Could you check a few things on this model? Use its own coordinates, in mm. A direction names the side the tool comes from. Round coordinates to 2 decimals unless told otherwise and drop trailing zeros. Write each loop counter-clockwise with the first axis right and the second up, starting at its lowest first coordinate (ties: lowest second). Pieces come first, ordered by that corner, then holes. Notation, with made-up numbers: (-21, 88) - (2, 88) arc R22 ccw to (2, 116) - close; hole circle Ø4 at (38, -12). An arc over 180 degrees is marked (long way). Write each question's results on one line, items separated by ' | '. Start each with the question number.
(1) Imagine slicing it at B-B on y = 24.5. Write out the boundary of the cut face in (x, z).
(2) Imagine slicing it at C-C on z = 0.5. Write out the boundary of the cut face in (x, y).
(3) Thinking about a two-plate mould opening in Y: for faces 4 (the flat face through (53, 82, 1)), 5 (the cylindrical face through (10.234, 71.195, 0.74)), 6 (the flat face through (109, 39, 1)), 7 (the flat face through (53, -2, 1)), which applies, +Y half, -Y half, draft (parallel to the pull), parting line (faces both ways), or undercut?
(4) Imagine slicing it at D-D on x = 37.5. Write out the boundary of the cut face in (y, z).
(5) Please list where these lines run through material, in increasing order: line 1 (Y direction, x = 11.04, z = 1.9); line 2 (X direction, y = 7.54, z = 1.9); line 3 (X direction, y = 58.5, z = 1.55). Write a range as [from, to].
(6) On a 3-axis mill with a long thin cutter (end or side, diameter ignored), from which of +Z, -Z, +X, -X, +Y, -Y can I reach the whole of each face in a straight line? I mean faces 1 (the flat face through (32, 5.8, 1)), 2 (the cylindrical face through (98.957, 7.408, 2.24)), 3 (the flat face through (-0.2, 40.2, 3)). Say none if no direction works.
(7) For P1, Ø3, axis at x = 97, y = 8, coming from the +Z side; P2, Ø2.5, axis at x = 11.04, y = 7.54, coming from the +Z side, each with a flat end and sliding along its axis, tell me the tip position at first contact or that it passes through.
(8) Imagine slicing it at A-A on x = 95.96. Write out the boundary of the cut face in (y, z), then the cut area to 3 significant figures.
```python
from build123d import *

# Parameters (mm, degrees)
SKETCH_9_W                                     = 111
SKETCH_9_H                                     = 84
BOTTOM_BASE_1P5MM_FULL_111X84_DEPTH            = 1.5
SKETCH_10_W                                    = 101
SKETCH_10_H                                    = 74
SKETCH_10_R                                    = 3
BOTTOM_CENTER_FULL_THICKNESS_EXCEPT_STAN_DEPTH = 3
SKETCH_11_W                                    = 111
SKETCH_11_H                                    = 2
BOTTOM_OUTER_FRONT_OVERHANG_FULL_3MM_DEPTH     = 3
SKETCH_12_W                                    = 111
SKETCH_12_H                                    = 2
BOTTOM_OUTER_REAR_OVERHANG_FULL_3MM_DEPTH      = 3
SKETCH_13_W                                    = 2
SKETCH_13_H                                    = 80
BOTTOM_OUTER_LEFT_OVERHANG_FULL_3MM_DEPTH      = 3
SKETCH_14_W                                    = 2
SKETCH_14_H                                    = 80
BOTTOM_OUTER_RIGHT_OVERHANG_FULL_3MM_DEPTH     = 3
SKETCH_16_R                                    = 1.5
BOTTOM_M3_THROUGH_3MM_DEPTH                    = 1.5
SKETCH_18_R                                    = 16.5
BOTTOM_BATTERY_THROUGH_CLEARANCE_DEPTH         = 3
SKETCH_20_W                                    = 23
SKETCH_20_H                                    = 23
BOTTOM_BUZZER_THROUGH_CUT_DEPTH                = 3


with BuildPart() as part:
    # Sketch 9 → bottom_base_1p5mm_full_111x84 (new body)
    with BuildSketch(Plane.XY):
        with Locations((53.5, 40)):
            Rectangle(SKETCH_9_W, SKETCH_9_H)
    extrude(amount=BOTTOM_BASE_1P5MM_FULL_111X84_DEPTH)

    # Sketch 10 → bottom_center_full_thickness_except_stan (add)
    with BuildSketch(Plane.XY):
        with Locations((53.5, 40)):
            Rectangle(SKETCH_10_W, SKETCH_10_H)
        with Locations(Location((11.04, 7.54, 0), (0, 0, 180))):
            Circle(SKETCH_10_R, mode=Mode.SUBTRACT)
        with Locations(Location((95.96, 7.54, 0), (0, 0, 180))):
            Circle(SKETCH_10_R, mode=Mode.SUBTRACT)
        with Locations(Location((11.04, 72.46, 0), (0, 0, 180))):
            Circle(SKETCH_10_R, mode=Mode.SUBTRACT)
        with Locations(Location((95.96, 72.46, 0), (0, 0, 180))):
            Circle(SKETCH_10_R, mode=Mode.SUBTRACT)
    extrude(amount=BOTTOM_CENTER_FULL_THICKNESS_EXCEPT_STAN_DEPTH)

    # Sketch 11 → bottom_outer_front_overhang_full_3mm (add)
    with BuildSketch(Plane.XY):
        with Locations((53.5, -1)):
            Rectangle(SKETCH_11_W, SKETCH_11_H)
    extrude(amount=BOTTOM_OUTER_FRONT_OVERHANG_FULL_3MM_DEPTH)

    # Sketch 12 → bottom_outer_rear_overhang_full_3mm (add)
    with BuildSketch(Plane.XY):
        with Locations((53.5, 81)):
            Rectangle(SKETCH_12_W, SKETCH_12_H)
    extrude(amount=BOTTOM_OUTER_REAR_OVERHANG_FULL_3MM_DEPTH)

    # Sketch 13 → bottom_outer_left_overhang_full_3mm (add)
    with BuildSketch(Plane.XY):
        with Locations((-1, 40)):
            Rectangle(SKETCH_13_W, SKETCH_13_H)
    extrude(amount=BOTTOM_OUTER_LEFT_OVERHANG_FULL_3MM_DEPTH)

    # Sketch 14 → bottom_outer_right_overhang_full_3mm (add)
    with BuildSketch(Plane.XY):
        with Locations((108, 40)):
            Rectangle(SKETCH_14_W, SKETCH_14_H)
    extrude(amount=BOTTOM_OUTER_RIGHT_OVERHANG_FULL_3MM_DEPTH)

    # Sketch 16 → bottom_m3_through_3mm (cut)
    with BuildSketch(Plane.XY):
        with Locations(Location((11.04, 7.54, 0), (0, 0, 180))):
            Circle(SKETCH_16_R)
        with Locations(Location((95.96, 7.54, 0), (0, 0, 180))):
            Circle(SKETCH_16_R)
        with Locations(Location((11.04, 72.46, 0), (0, 0, 180))):
            Circle(SKETCH_16_R)
        with Locations(Location((95.96, 72.46, 0), (0, 0, 180))):
            Circle(SKETCH_16_R)
    extrude(amount=BOTTOM_M3_THROUGH_3MM_DEPTH, mode=Mode.SUBTRACT)

    # Sketch 18 → bottom_battery_through_clearance (cut)
    with BuildSketch(Plane.XY):
        with Locations(Location((58.8, 24.5, 0), (0, 0, 180))):
            Circle(SKETCH_18_R)
    extrude(amount=BOTTOM_BATTERY_THROUGH_CLEARANCE_DEPTH, mode=Mode.SUBTRACT)

    # Sketch 20 → bottom_buzzer_through_cut (cut)
    with BuildSketch(Plane.XY):
        with Locations((32.4, 17.3)):
            Rectangle(SKETCH_20_W, SKETCH_20_H)
    extrude(amount=BOTTOM_BUZZER_THROUGH_CUT_DEPTH, mode=Mode.SUBTRACT)


solid = part.part
```
Response:
1) outline: (-2, 0) - (20.9, 0) - (20.9, 3) - (3, 3) - (3, 1.5) - (0, 1.5) - (0, 3) - (-2, 3) - close; (75.3, 0) - (109, 0) - (109, 3) - (107, 3) - (107, 1.5) - (104, 1.5) - (104, 3) - (75.3, 3) - close
2) outline: (-2, -2) - (109, -2) - (109, 82) - (-2, 82) - close; hole circle Ø3 at (11.04, 7.54); hole circle Ø3 at (11.04, 72.46); hole (20.9, 5.8) - (43.9, 5.8) - (43.9, 17.41) arc R16.5 ccw (long way) to (42.87, 28.8) - (20.9, 28.8) - close; hole circle Ø3 at (95.96, 7.54); hole circle Ø3 at (95.96, 72.46)
3) face 4: +Y half | face 5: undercut | face 6: draft | face 7: -Y half
4) outline: (-2, 0) - (5.8, 0) - (5.8, 3) - (3, 3) - (3, 1.5) - (0, 1.5) - (0, 3) - (-2, 3) - close; (28.8, 0) - (82, 0) - (82, 3) - (80, 3) - (80, 1.5) - (77, 1.5) - (77, 3) - (28.8, 3) - close
5) line 1: [-2, 0], [3, 4.54], [10.54, 69.46], [75.46, 77], [80, 82] | line 2: [-2, 0], [3, 8.04], [14.04, 20.9], [43.9, 92.96], [98.96, 104], [107, 109] | line 3: [-2, 0], [3, 104], [107, 109]
6) face 1: +Z, -Z | face 2: +Z | face 3: +Z, +X, -X, +Y, -Y
7) P1: z = 1.5 | P2: through
8) outline: (-2, 0) - (6.04, 0) - (6.04, 1.5) - (4.54, 1.5) - (4.54, 3) - (3, 3) - (3, 1.5) - (0, 1.5) - (0, 3) - (-2, 3) - close; (9.04, 0) - (70.96, 0) - (70.96, 1.5) - (69.46, 1.5) - (69.46, 3) - (10.54, 3) - (10.54, 1.5) - (9.04, 1.5) - close; (73.96, 0) - (82, 0) - (82, 3) - (80, 3) - (80, 1.5) - (77, 1.5) - (77, 3) - (75.46, 3) - (75.46, 1.5) - (73.96, 1.5) - close | area: 216 mm²
